Autodesk Inventor part; units mm, degrees
ref_plane "YZ Plane" through (0, 0, 0) normal (1, 0, 0) x (0, 1, 0)
ref_plane "XZ Plane" through (0, 0, 0) normal (0, 1, 0) x (-1, 0, 0)
ref_plane "XY Plane" through (0, 0, 0) normal (0, 0, 1) x (1, 0, 0)
sketch "Эскиз1" plane through (0, 0, 0) normal (0, 0, 1) x (1, 0, 0)
  circle A0 centre (0, 0) radius 4.5
  line L0 (-9, -4) -> (-20, -4)
  line L1 (-20, -4) -> (-20, -5)
  line L2 (20, -5) -> (20, -4)
  line L3 (20, -4) -> (9, -4)
  line L4 (-20, -5) -> (-20, -7)
  line L5 (-20, -7) -> (20, -7)
  line L6 (20, -7) -> (20, -5)
  arc A1 (7, 0) -> (-7, 0) centre (0, 0) ccw
  line L7 (-7, 0) -> (-7, -2)
  line L8 (7, 0) -> (7, -2)
  arc A2 (-9, -4) -> (-7, -2) centre (-9, -2) ccw
  arc A3 (7, -2) -> (9, -4) centre (9, -2) ccw
  point P0 (3, -4)
  point P1 (-5, 0)
  point P2 (-5, -4)
  point P3 (5, 0)
  point P4 (5, -4)
  dimension "d0" = 9
  dimension "d2" = 1
  dimension "d20" = 2
  dimension "d21" = 14
  dimension "d22" = 2
extrude "Выдавливание4" add sketch "Эскиз1" along normal blind 50
sketch "Эскиз3" plane through (9, -4, 0) normal (0, 1, 0) x (1, 0, 0)
  circle A0 centre (-21.4987, -10) radius 1.5
  circle A1 centre (-21.4987, -25) radius 1.5
  circle A2 centre (-21.4987, -40) radius 1.5
  circle A3 centre (3.5013, -10) radius 1.5
  circle A4 centre (3.5013, -25) radius 1.5
  circle A5 centre (3.5013, -40) radius 1.5
  line L0 (5.2423, -9.8461) -> (4.5051, -11.4308)
  line L1 (4.5051, -11.4308) -> (2.7641, -11.5846)
  line L2 (2.7641, -11.5846) -> (1.7604, -10.1539)
  line L3 (1.7604, -10.1539) -> (2.4976, -8.5692)
  line L4 (2.4976, -8.5692) -> (4.2386, -8.4154)
  line L5 (4.2386, -8.4154) -> (5.2423, -9.8461)
  line L6 (2.3986, -8.2924) -> (4.4288, -8.1912)
  line L7 (4.4288, -8.1912) -> (5.5315, -9.8988)
  line L8 (5.5315, -9.8988) -> (4.604, -11.7076)
  line L9 (4.604, -11.7076) -> (2.5739, -11.8088)
  line L10 (2.5739, -11.8088) -> (1.4712, -10.1012)
  line L11 (1.4712, -10.1012) -> (2.3986, -8.2924)
  line L12 (3.5013, -10) -> (2.0013, -10)
  line L13 (3.5013, -10) -> (3.5013, -11.5)
  line L14 (1.4712, -25.1012) -> (2.3986, -23.2924)
  line L15 (2.3986, -23.2924) -> (4.4288, -23.1912)
  line L16 (4.4288, -23.1912) -> (5.5315, -24.8988)
  line L17 (4.2386, -23.4154) -> (5.2423, -24.8461)
  line L18 (2.4976, -23.5692) -> (4.2386, -23.4154)
  line L19 (1.7604, -25.1539) -> (2.4976, -23.5692)
  line L20 (2.7641, -26.5846) -> (1.7604, -25.1539)
  line L21 (2.5739, -26.8088) -> (1.4712, -25.1012)
  line L22 (4.604, -26.7076) -> (2.5739, -26.8088)
  line L23 (4.5051, -26.4308) -> (2.7641, -26.5846)
  line L24 (5.2423, -24.8461) -> (4.5051, -26.4308)
  line L25 (5.5315, -24.8988) -> (4.604, -26.7076)
  line L26 (1.4712, -40.1012) -> (2.3986, -38.2924)
  line L27 (2.3986, -38.2924) -> (4.4288, -38.1912)
  line L28 (4.4288, -38.1912) -> (5.5315, -39.8988)
  line L29 (4.2386, -38.4154) -> (5.2423, -39.8461)
  line L30 (2.4976, -38.5692) -> (4.2386, -38.4154)
  line L31 (1.7604, -40.1539) -> (2.4976, -38.5692)
  line L32 (2.7641, -41.5846) -> (1.7604, -40.1539)
  line L33 (2.5739, -41.8088) -> (1.4712, -40.1012)
  line L34 (4.604, -41.7076) -> (2.5739, -41.8088)
  line L35 (4.5051, -41.4308) -> (2.7641, -41.5846)
  line L36 (5.2423, -39.8461) -> (4.5051, -41.4308)
  line L37 (5.5315, -39.8988) -> (4.604, -41.7076)
  line L38 (-23.5288, -10.1012) -> (-22.6014, -8.2924)
  line L39 (-22.6014, -8.2924) -> (-20.5712, -8.1912)
  line L40 (-20.5712, -8.1912) -> (-19.4685, -9.8988)
  line L41 (-20.7614, -8.4154) -> (-19.7577, -9.8461)
  line L42 (-22.5024, -8.5692) -> (-20.7614, -8.4154)
  line L43 (-23.2396, -10.1539) -> (-22.5024, -8.5692)
  line L44 (-22.2359, -11.5846) -> (-23.2396, -10.1539)
  line L45 (-22.4261, -11.8088) -> (-23.5288, -10.1012)
  line L46 (-20.396, -11.7076) -> (-22.4261, -11.8088)
  line L47 (-20.4949, -11.4308) -> (-22.2359, -11.5846)
  line L48 (-19.7577, -9.8461) -> (-20.4949, -11.4308)
  line L49 (-19.4685, -9.8988) -> (-20.396, -11.7076)
  line L50 (-23.5288, -25.1012) -> (-22.6014, -23.2924)
  line L51 (-22.6014, -23.2924) -> (-20.5712, -23.1912)
  line L52 (-20.5712, -23.1912) -> (-19.4685, -24.8988)
  line L53 (-20.7614, -23.4154) -> (-19.7577, -24.8461)
  line L54 (-22.5024, -23.5692) -> (-20.7614, -23.4154)
  line L55 (-23.2396, -25.1539) -> (-22.5024, -23.5692)
  line L56 (-22.2359, -26.5846) -> (-23.2396, -25.1539)
  line L57 (-22.4261, -26.8088) -> (-23.5288, -25.1012)
  line L58 (-20.396, -26.7076) -> (-22.4261, -26.8088)
  line L59 (-20.4949, -26.4308) -> (-22.2359, -26.5846)
  line L60 (-19.7577, -24.8461) -> (-20.4949, -26.4308)
  line L61 (-19.4685, -24.8988) -> (-20.396, -26.7076)
  line L62 (-23.5288, -40.1012) -> (-22.6014, -38.2924)
  line L63 (-22.6014, -38.2924) -> (-20.5712, -38.1912)
  line L64 (-20.5712, -38.1912) -> (-19.4685, -39.8988)
  line L65 (-20.7614, -38.4154) -> (-19.7577, -39.8461)
  line L66 (-22.5024, -38.5692) -> (-20.7614, -38.4154)
  line L67 (-23.2396, -40.1539) -> (-22.5024, -38.5692)
  line L68 (-22.2359, -41.5846) -> (-23.2396, -40.1539)
  line L69 (-22.4261, -41.8088) -> (-23.5288, -40.1012)
  line L70 (-20.396, -41.7076) -> (-22.4261, -41.8088)
  line L71 (-20.4949, -41.4308) -> (-22.2359, -41.5846)
  line L72 (-19.7577, -39.8461) -> (-20.4949, -41.4308)
  line L73 (-19.4685, -39.8988) -> (-20.396, -41.7076)
  point P0 (-9, 0)
  dimension "d51" = 15
  dimension "d54" = 25
extrude "Выдавливание5" cut sketch "Эскиз3" against normal blind 3 contours A0
extrude "Выдавливание6" cut sketch "Эскиз3" against normal blind 3 contours A1 | A2 | A3 L13 L12 | L12 L13 A3 | A4 | A5
extrude "Выдавливание7" add sketch "Эскиз3" along normal blind 2 contours L6 L7 L8 L9 L10 L11 | L14 L15 L16 L25 L22 L21 | L26 L27 L28 L37 L34 L33 | L38 L39 L40 L49 L46 L45 | L50 L51 L52 L61 L58 L57 | L62 L63 L64 L73 L70 L69
properties part number "крепление направляющей руки"
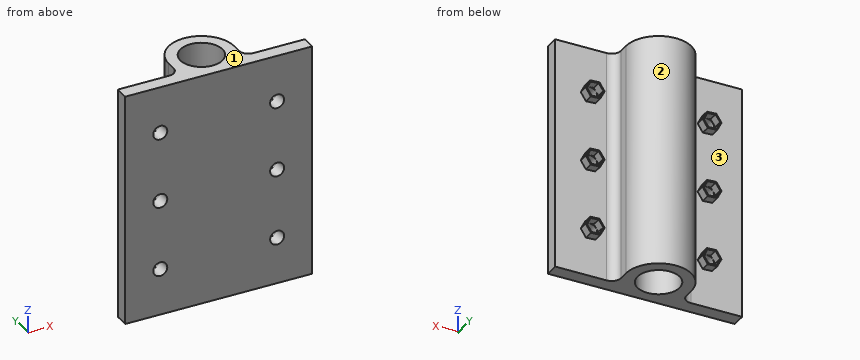
Work out the finished part from the listing and answer in its coordinate system (mm). Face numbers are marked on the shaded views. Give positions to 0.01 mm unless a question says otherwise; leave off trailing zeros. Loops run counter-clockwise (first coordinate to the right, second up) from the corner with the lowest first, then second, coordinate; pieces in that order, holes last. Notation, with made-up numbers: (-10, -39.5) - (48, -39.5) arc R20 ccw to (48, -4.5) - close; hole circle Ø5 at (65, 65.25). An arc over 180 degrees is marked (long way). Answer in a Markdown table with one row per item. Add a question column.
Q1. The part is cut by section B-B (z = 45). Determine the outline of the cut face in (x, y), and give its area (3 significant figures).
Q2. The part is cut by section A-A (y = 1.5). Determine the outline of the cut face in (x, z).
Q3. Consider line 1 along X through (y, z) = (-6.3, 10); line 2 along X through (y, z) = (-6, 24); line 3 along Y through (x, z) = (0, 25). Determine where each line is inside the solid, lowest interval first.
Q4. Each of these flat-tipped pins is pushed along its axis until it touches: P1, Ø1, axis at x = -13.5, z = 24.5, coming from the +Y side; P2, Ø8, axis at y = 3.5, z = 34, coming from the -X side; P3, Ø2.5, axis at x = 12.5, z = 25, coming from the -Y side; P4, Ø2, axis at x = 2.5, z = 36, coming from the +Y side. Where does it stop, or does it pass through?
Q5. Determine the mould class of the marked faces 1, 2 and 3 for opening direction Z: released by +Z, released by -Z, zero draft, split by the parting line, or undercut.
Q6. The part is cut by section C-C (x = 12.5). State how many separate pieces and enclosed holes the cut face has, and give its area (3 significant figures).
Solution:
| question | item | result |
|---|---|---|
| 1 | outline | (-20, -7) - (20, -7) - (20, -4) - (9, -4) arc R2 cw to (7, -2) - (7, 0) arc R7 ccw to (-7, 0) - (-7, -2) arc R2 cw to (-9, -4) - (-20, -4) - close; hole circle Ø9 at (0, 0) |
| 1 | area | 191 mm² |
| 2 | outline | (-6.84, 0) - (-4.24, 0) - (-4.24, 50) - (-6.84, 50) - close; (4.24, 0) - (6.84, 0) - (6.84, 50) - (4.24, 50) - close |
| 3 | line 1 | x = -20 to -14, -11 to 11, 14 to 20 |
| 3 | line 2 | x = -20 to -13.62, -11.38 to 11.38, 13.62 to 20 |
| 3 | line 3 | y = -7 to -4.5, 4.5 to 7 |
| 4 | P1 | stops at y = -2 |
| 4 | P2 | stops at x = -7 |
| 4 | P3 | passes through |
| 4 | P4 | stops at y = 6.84 |
| 5 | face 1 | released by +Z |
| 5 | face 2 | zero draft |
| 5 | face 3 | undercut |
| 6 | separate pieces | 4 |
| 6 | enclosed holes | 0 |
| 6 | area | 126 mm² |
